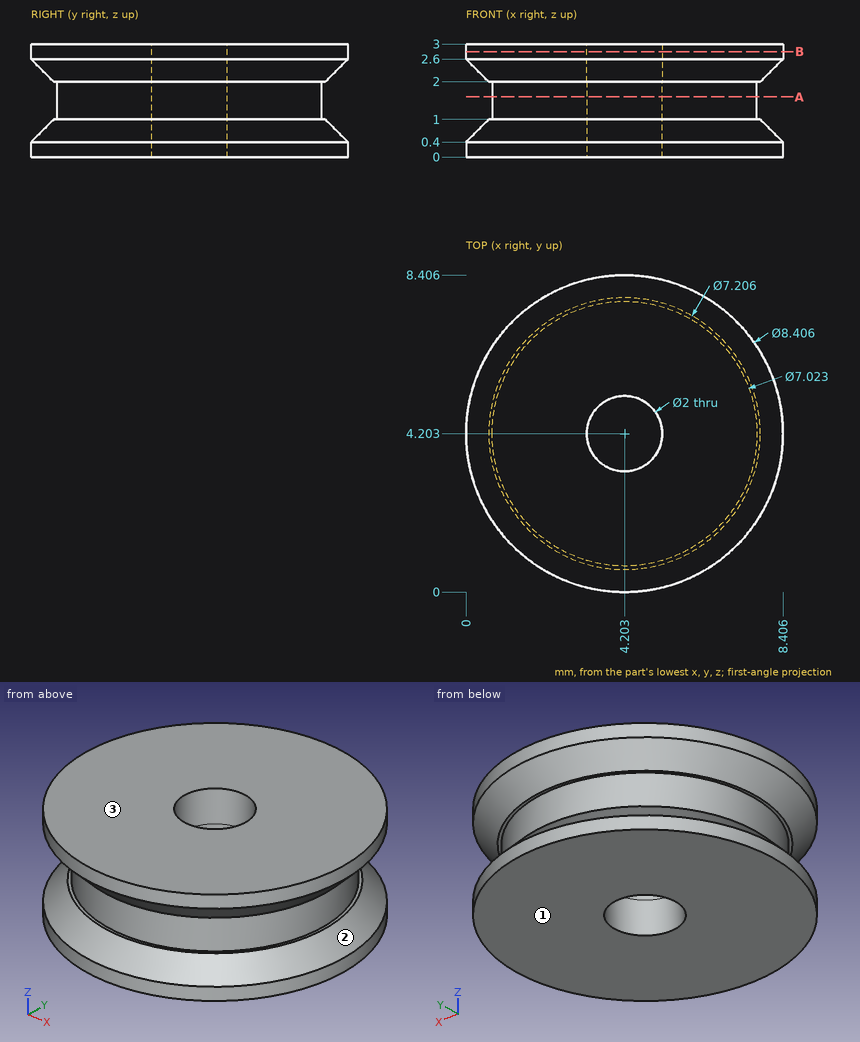
Check sheet for the drawn part. Datum: minimum x, y, z corner. Units: mm. Round coordinates to 2 decimals unless told otherwise and drop trailing zeros. Order: outer loops, then holes, each group sorted by start corner. A loop starts at its lowest first (then second) coordinate and runs counter-clockwise, first axis right, second up.
(1) Cross-section at B-B, the plane z = 2.8. Enter the section's corners in (x, y) (1 decimal).
(2) Go/stop test with flat-tipped pins: P1, Ø1.2, axis at x = 4.2, y = 4.2, coming from the -Z side; P2, Ø1, axis at x = 3.5, z = 2, coming from the -Y side (1 decimal). Record where each tip stops, or that it passes through.
(3) Draft check along Z on the marked faces 1, 2 and 3. Enter one of: pulls with the +Z half, pulls with the -Z half, needs draft (parallel to the pull), parting line crosses it, or undercut.
(4) Cross-section at A-A, the plane z = 1.6. Enter the section's corners in (x, y).
(5) Scan lines: probe 1 along X at (y, z) = (4.25, 1.3); probe 2 along Z at (x, y) = (7.75, 3.75); probe 3 along Y at (x, z) = (5, 1.1) (1 decimal). Record each from-to range of solid material in increasing order.
Check sheet entries:
1. outline: circle Ø8.4 at (4.2, 4.2); hole circle Ø2 at (4.2, 4.2)
2. P1: passes through
2. P2: stops at y = 0.2
3. face 1: pulls with the -Z half
3. face 2: undercut
3. face 3: pulls with the +Z half
4. outline: circle Ø7.02 at (4.2, 4.2); hole circle Ø2 at (4.2, 4.2)
5. probe 1: x = 0.69 to 3.2, 5.2 to 7.71
5. probe 2: z = 0 to 1, 2 to 3
5. probe 3: y = 0.8 to 3.6, 4.8 to 7.6
